Part model, mm, in its own coordinate system. Face numbers are marked on the shaded views. A direction names the side the tool comes from. Give positions to 0.01 mm unless a question says otherwise; leave off trailing zeros. Write each loop counter-clockwise with the first axis right and the second up, starting at its lowest first coordinate (ties: lowest second). Pieces come first, ordered by that corner, then holes. Notation, with made-up numbers: M -14.75,87.5 L -9.75,87.5 A23 cw -9.75,110.5 Z; hole C 13,70 d1. An arc over 180 degrees is marked long. Use a Markdown table: item, result.
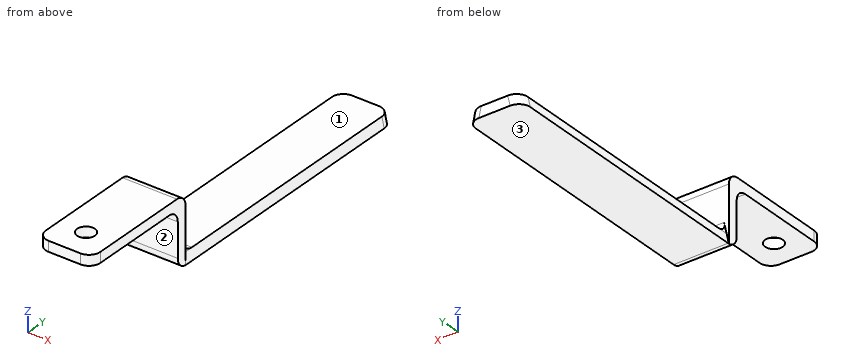
```python
from build123d import *

# Parameters (mm, degrees)
F1_DEPTH      = 127
F2_W          = 24.3321505244
F2_H          = 4.6101
F3_DEPTH      = 25.4
F3_DEPTH_BACK = 4.6101
F4_W          = 24.3321505244
F4_H          = 4.6101
F5_DEPTH      = 50.8
F6_T1_DEPTH   = 24.3321505244
F6_T6_DEPTH   = 47.6747505244
F6_T9_DEPTH   = 49.7321505244
F6_T11_DEPTH  = 30.0101
F6_T13_DEPTH  = 30.1234781359
F6_T15_DEPTH  = 30.1234781359
F8_D          = 7.9375
F8_DEPTH      = 19.05
F8_TIP        = 2.3846655818


# Not quite as in the source:
# - a fillet or chamfer that OpenCascade refuses, or shapes differently, is made with other operations: its cross-section is extruded or revolved along the edge and cut away or added


with BuildPart() as f1:
    # F0 (on Front) → F1 (new body)
    with BuildSketch(Plane.XZ):
        Polygon((1.8483747378, 4.6101), (0.8196747378, 0), (25.1518252622, 0), (24.1231252622, 4.6101), align=None)
    extrude(amount=F1_DEPTH)

    # F2 (on face) → F3 (join, two sides)
    with BuildSketch(Plane.XY.offset(4.6101)) as f3_sk:
        with Locations((12.98575, -124.69495)):
            Rectangle(F2_W, F2_H)
    extrude(amount=F3_DEPTH)
    extrude(f3_sk.sketch, amount=-F3_DEPTH_BACK)

    # F4 (on face) → F5 (join)
    with BuildSketch(Plane.XZ.offset(127)):
        with Locations((12.98575, 27.70505)):
            Rectangle(F4_W, F4_H)
    extrude(amount=F5_DEPTH)

    # F6: fillet of radius 5.08 on 8 edges, made by hand

    # F6_s2 → F6_t1 (join)
    with BuildSketch(Plane.YZ.offset(0.8196747378)):
        with BuildLine():
            ThreePointArc((-132.08, 25.4), (-128.4878975516, 23.9121024484), (-127, 20.32))
            Line((-127, 20.32), (-127, 25.4))
            Line((-127, 25.4), (-132.08, 25.4))
        make_face()
    extrude(amount=F6_T1_DEPTH)


with BuildPart() as f6_tool4:
    # F6_s5 → F6_t6 (new body)
    with BuildSketch(Plane.YZ.offset(36.8231252622)):
        with BuildLine():
            ThreePointArc((-117.3099, 4.6101), (-120.9020024484, 6.0979975516), (-122.3899, 9.6901))
            Line((-122.3899, 9.6901), (-122.3899, 4.6101))
            Line((-122.3899, 4.6101), (-117.3099, 4.6101))
        make_face()
    extrude(amount=-F6_T6_DEPTH)

    split(bisect_by=Plane(origin=(0.780797517, 0, -0.1742275451), x_dir=(0, 1, 0), z_dir=(0.9759968962, 0, -0.2177844314)), keep=Keep.TOP)

    split(bisect_by=Plane(origin=(23.9588727172, 0, 5.3461947386), x_dir=(0, 1, 0), z_dir=(-0.9759968962, 0, -0.2177844314)), keep=Keep.TOP)


with BuildPart() as f1_1:
    add(f1.part)

    # F6_t3: union F6_tool4
    add(f6_tool4.part)

    # F6_s10 → F6_t9 (cut)
    with BuildSketch(Plane.YZ.offset(-11.8803252622)):
        with BuildLine():
            ThreePointArc((-127.4699, 30.0101), (-123.8777975516, 28.5222024484), (-122.3899, 24.9301))
            Line((-122.3899, 24.9301), (-122.3899, 30.0101))
            Line((-122.3899, 30.0101), (-127.4699, 30.0101))
        make_face()
        with BuildLine():
            ThreePointArc((-121.92, 0), (-125.5121024484, 1.4878975516), (-127, 5.08))
            Line((-127, 5.08), (-127, 0))
            Line((-127, 0), (-121.92, 0))
        make_face()
    extrude(amount=F6_T9_DEPTH, mode=Mode.SUBTRACT)

    # F6_s12 → F6_t11 (cut)
    with BuildSketch(Plane.XY.offset(12.7)):
        with BuildLine():
            ThreePointArc((5.8996747378, -177.8), (2.3075722894, -176.3121024484), (0.8196747378, -172.72))
            Line((0.8196747378, -172.72), (0.8196747378, -177.8))
            Line((0.8196747378, -177.8), (5.8996747378, -177.8))
        make_face()
        with BuildLine():
            ThreePointArc((25.1518252622, -172.72), (23.6639277106, -176.3121024484), (20.0718252622, -177.8))
            Line((20.0718252622, -177.8), (25.1518252622, -177.8))
            Line((25.1518252622, -177.8), (25.1518252622, -172.72))
        make_face()
    extrude(amount=F6_T11_DEPTH, mode=Mode.SUBTRACT)

    # F6_s14 → F6_t13 (cut)
    with BuildSketch(Plane(origin=(3.8334394995, 0, 17.1794881272), x_dir=(0, 1, 0), z_dir=(-0.2177844314, 0, -0.9759968962))):
        with BuildLine():
            ThreePointArc((-5.08, 0.8), (-1.4878975516, 2.2878975516), (0, 5.88))
            Line((0, 5.88), (0, 0.8))
            Line((0, 0.8), (-5.08, 0.8))
        make_face()
    extrude(amount=F6_T13_DEPTH, mode=Mode.SUBTRACT)

    # F6_s16 → F6_t15 (cut)
    with BuildSketch(Plane(origin=(3.9588148236, 0, -17.7413553206), x_dir=(0, 1, 0), z_dir=(-0.2177844314, 0, 0.9759968962))):
        with BuildLine():
            ThreePointArc((-5.08, -24.5481033904), (-1.4878975516, -23.0602058388), (0, -19.4681033904))
            Line((0, -19.4681033904), (0, -24.5481033904))
            Line((0, -24.5481033904), (-5.08, -24.5481033904))
        make_face()
    extrude(amount=F6_T15_DEPTH, mode=Mode.SUBTRACT)

    # F8
    with Locations(Plane.XY.offset(30.0101)):
        with Locations((12.98575, -165.1)):
            Hole(F8_D / 2, depth=F8_DEPTH)
            with Locations((0, 0, -(F8_DEPTH + F8_TIP / 2))):  # 118° drill point
                Cone(0, F8_D / 2, F8_TIP, mode=Mode.SUBTRACT)


solid = f1_1.part
```
1. Cut at C-C, the plane z = 28. Give the cut face in (x, y), then the cut area to 3 significant figures.
Findings below:
| item | result |
|---|---|
| outline | M 0.82,-172.72 A5.08 ccw 5.9,-177.8 L 20.07,-177.8 A5.08 ccw 25.15,-172.72 L 25.15,-123.42 L 0.82,-123.42 Z; hole C 12.99,-165.1 d7.94 |
| area | 1,260 mm2 |
2. Drill centre lines: L1, parallel to X at y = -165, z = 27; L2, parallel to Z at x = 9.5, y = -36.5; L3, parallel to Z at x = 17.25, y = -169. Where is each one in solid material? Low to high.
Findings below:
| item | result |
|---|---|
| L1 | 0.82 to 9.02, 16.95 to 25.15 |
| L2 | 0 to 4.61 |
| L3 | 25.4 to 30.01 |
3. Tool access for the marked faces 1, 2 and 3: list every direction of +Z, -Z, +X, -X, +Y, -Y with a clear straight run to the whole face (end or side of a thin tool).
Findings below:
| item | result |
|---|---|
| face 1 | +Z, +X, -X, +Y |
| face 2 | -Z, +X, -X, -Y |
| face 3 | -Z, +X, -X, +Y, -Y |
4. Cut at D-D, the plane y = -16.5. Give the cut face in (x, z), then the cut area to 3 significant figures.
Findings below:
| item | result |
|---|---|
| outline | M 0.82,0 L 25.15,0 L 24.12,4.61 L 1.85,4.61 Z |
| area | 107 mm2 |
5. Cut at B-B, the plane x = 11. Give the cut face in (y, z), then the cut area to 3 significant figures.
Findings below:
| item | result |
|---|---|
| outline | M -177.8,25.4 L -168.54,25.4 L -168.54,30.01 L -177.8,30.01 Z; M -161.66,25.4 L -132.08,25.4 A5.08 cw -127,20.32 L -127,5.08 A5.08 ccw -121.92,0 L 0,0 L 0,4.61 L -117.31,4.61 A5.08 cw -122.39,9.69 L -122.39,24.93 A5.08 ccw -127.47,30.01 L -161.66,30.01 Z |
| area | 905 mm2 |
6. Cut at A-A, the plane y = -165.1. Give the cut face in (x, z), then the cut area to 3 significant figures.
Findings below:
| item | result |
|---|---|
| outline | M 0.82,25.4 L 9.02,25.4 L 9.02,30.01 L 0.82,30.01 Z; M 16.95,25.4 L 25.15,25.4 L 25.15,30.01 L 16.95,30.01 Z |
| area | 75.6 mm2 |
7. Drop flat-ended pins along their axis: P1, Ø3, axis at x = 21, z = 24, coming from the +Y side; P2, Ø3, axis at y = -133.5, z = 22, coming from the -X side; P3, Ø10.5, axis at x = 12.99, y = -165.1, coming from the -Z side; P4, Ø1, axis at x = 11.5, y = -112, coming from the +Z side. Give the stop position or say it passes through.
Findings below:
| item | result |
|---|---|
| P1 | y = -122.39 |
| P2 | through |
| P3 | z = 25.4 |
| P4 | z = 4.61 |
